Source: three-view drawing plus pictorial views. Frame: mm from the lowest corner of the part. A direction names the side the tool comes from. Give positions to 0.01 mm unless a question says otherwise; leave off trailing zeros. Loops run counter-clockwise (first coordinate to the right, second up) from the corner with the lowest first, then second, coordinate; pieces in that order, holes last.
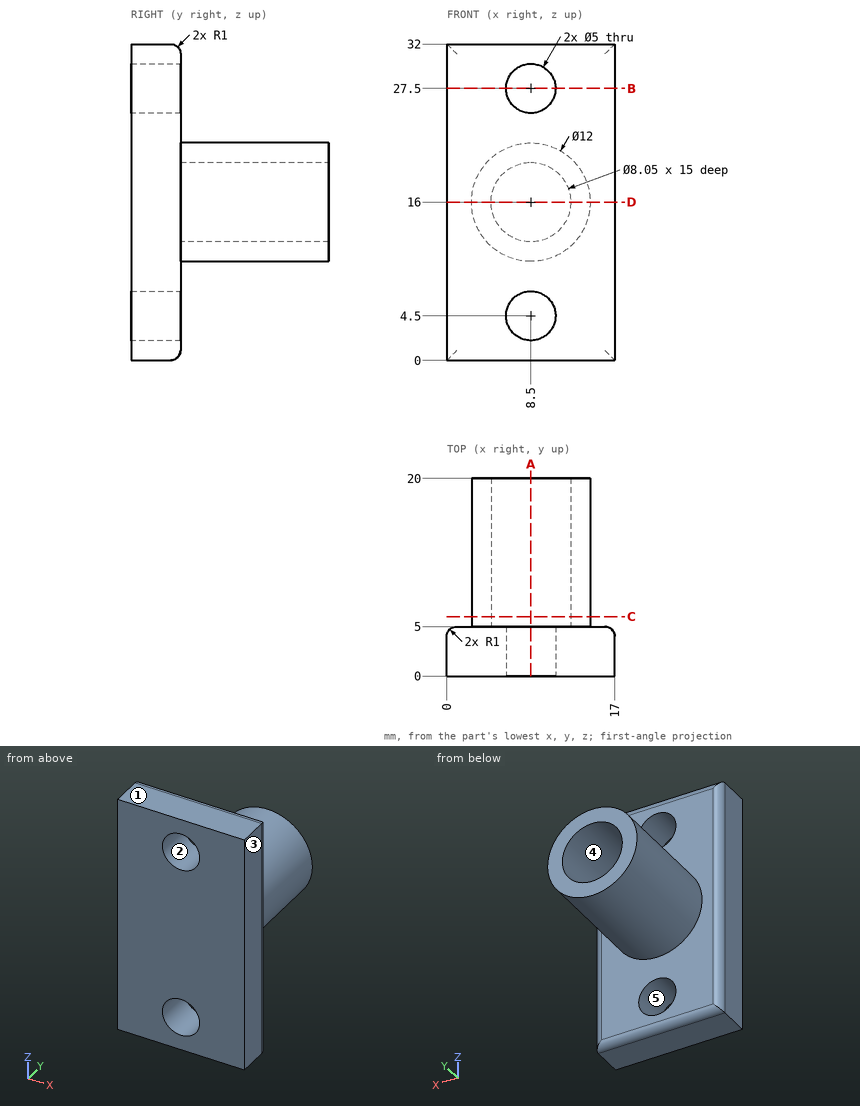
1) Cut plane C-C (y = 6). Return loops of the section in (x, z) (3 decimals).
Checks:
outline: circle Ø12 at (8.5, 16); hole circle Ø8.05 at (8.5, 16)
2) Cut plane D-D (z = 16). Return loops of the section in (x, y) (3 decimals).
Checks:
outline: (0, 0) - (17, 0) - (17, 4) arc R1 ccw to (16, 5) - (14.5, 5) - (14.5, 20) - (12.525, 20) - (12.525, 5) - (4.475, 5) - (4.475, 20) - (2.5, 20) - (2.5, 5) - (1, 5) arc R1 ccw to (0, 4) - close
3) Cut plane B-B (z = 27.5). Return loops of the section in (x, y), and give its area (3 significant figures).
Checks:
outline: (0, 0) - (6, 0) - (6, 5) - (1, 5) arc R1 ccw to (0, 4) - close; (11, 0) - (17, 0) - (17, 4) arc R1 ccw to (16, 5) - (11, 5) - close
area: 59.6 mm2
4) Ray query, probe 1 along Z at (x, y) = (7.25, 4.5); probe 2 along X at (y, z) = (9.25, 16) (3 decimals); probe 3 along Y at (x, z) = (12, 9.5). Return the intervals inside material, ascending.
Checks:
probe 1: z = 0.13 to 2.33, 6.67 to 25.33, 29.67 to 31.87
probe 2: x = 2.5 to 4.475, 12.525 to 14.5
probe 3: y = 0 to 5
5) Contact query for flat-ended pins moving along their axis: P1, Ø8, axis at y = 17.5, z = 8.5, coming from the -X side; P2, Ø6, axis at x = 11, z = 27, coming from the +Y side; P3, Ø6.5, axis at x = 8.5, z = 4.5, coming from the -Y side; P4, Ø2, axis at y = 14, z = 17, coming from the -X side. Output: stop coordinate, or through.
Checks:
P1: stops at x = 3.63
P2: stops at y = 5
P3: stops at y = 0
P4: stops at x = 2.5
6) Reachability of the marked faces 4 and 5 from +Z, -Z, +X, -X, +Y, -Y: full face, straight path, thin tool, end or side. Return the list, or none.
Checks:
face 4: +Y
face 5: +Y, -Y
7) Pull-direction query (Z, two-part tool) for the marked faces 1, 2 and 3; classes: released by +Z, released by -Z, zero draft, split by the parting line, or undercut.
Checks:
face 1: released by +Z
face 2: undercut
face 3: zero draft
8) Cut plane A-A (x = 8.5). Return loops of the section in (y, z) (3 decimals).
Checks:
outline: (0, 0) - (4, 0) arc R1 ccw to (5, 1) - (5, 2) - (0, 2) - close; (0, 7) - (5, 7) - (5, 10) - (20, 10) - (20, 11.975) - (5, 11.975) - (5, 20.025) - (20, 20.025) - (20, 22) - (5, 22) - (5, 25) - (0, 25) - close; (0, 30) - (5, 30) - (5, 31) arc R1 ccw to (4, 32) - (0, 32) - close
